For this review, use the dimensioned drawing (mm, ordinates from the lowest corner) and the shaded views. Coordinates: 2 decimals unless noted, no trailing zeros. Use CSV: the item, a comma, the result in double quotes.
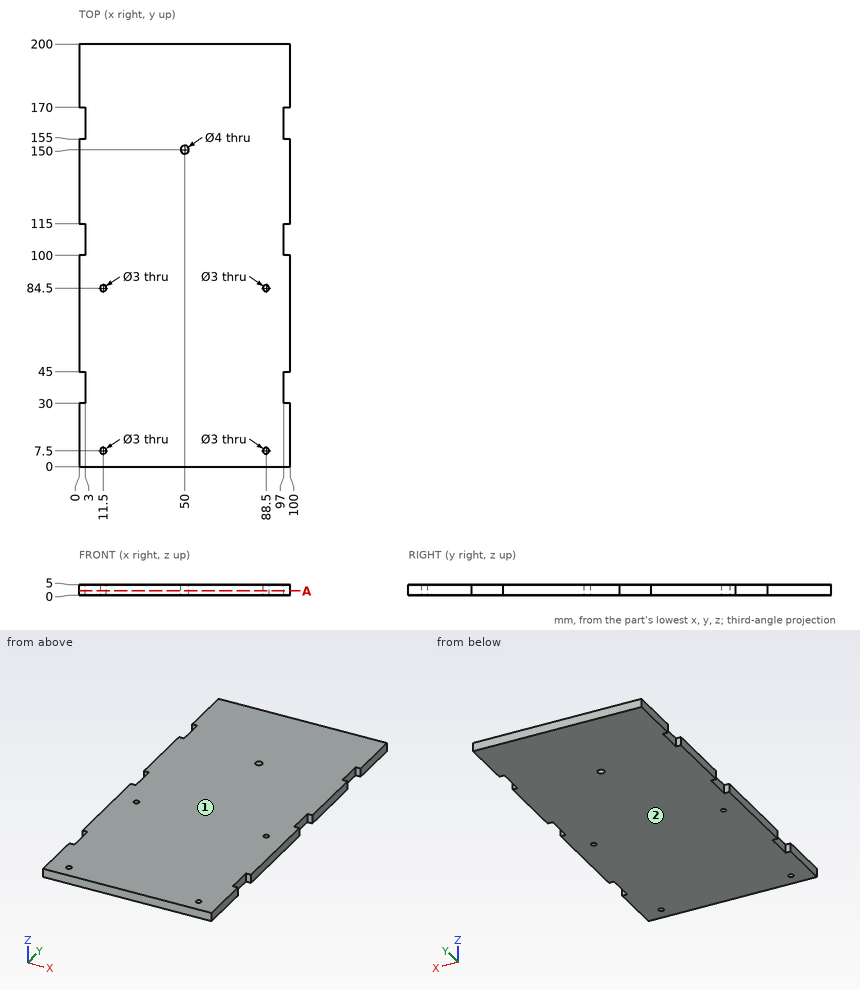
Item 1: To check wall thickness, follow line 1 along Y through (x, z) = (88.5, 3.15); line 2 along X through (y, z) = (7.5, 3.75); line 3 along X through (y, z) = (161, 3.8). State the ranges of each line that lie inside material, in increasing order. Write a range as [from, to].
Solutions:
line 1,"[0, 6], [9, 83], [86, 200]"
line 2,"[0, 10], [13, 87], [90, 100]"
line 3,"[3, 97]"
Item 2: Add section A-A on z = 2.1. State how many separate pieces and enclosed holes the cut face has, and give its area (3 significant figures).
Solutions:
separate pieces,"1"
enclosed holes,"5"
area,"19,700 mm^2"
Item 3: Clearance check with flat-ended pins moving along their axes: pin 1 Ø1.5 at (x, z) = (1, 2.5) entering from -Y; pin 2 Ø2.5 at (y, z) = (107, 1.5) entering from +X; pin 3 Ø2.5 at (y, z) = (159.5, 1.5) entering from -X. State where each tip first meets the part, or that it passes through.
Solutions:
pin 1,"y = 0"
pin 2,"x = 97"
pin 3,"x = 3"
Item 4: Draft analysis for pull direction Z (two halves, no side actions). For the marked faces 1 and 2, state which applies: released by +Z, released by -Z, zero draft, split by the parting line, or undercut.
Solutions:
face 1,"released by +Z"
face 2,"released by -Z"
